```python
from build123d import *

# Parameters (mm, degrees)
F1_DEPTH = 63.5
F2_DEPTH = 3.175
F0_W     = 22.2610938409
F0_H     = 19.05
F3_DEPTH = 25.4
F5_DEPTH = 25.4
F6_R     = 6.35


with BuildPart() as f1:
    # F0 (on Front) → F1 (new body, symmetric)
    with BuildSketch(Plane.XZ):
        Polygon((-41.275, 9.525), (-41.275, -9.525), (41.275, -9.525), (41.275, 9.525), (22.225, 9.525), align=None)
    extrude(amount=F1_DEPTH, both=True)

    # F0 (on Front) → F2 (join, symmetric)
    with BuildSketch(Plane.XZ):
        with BuildLine():
            add(Edge.make_bspline(
                [(-41.275, 9.525), (-34.2779420316, 38.2648594677), (15.5508974567, 65.6356289983), (57.15, 61.9252)],
                knots=[0, 0, 0, 0, 111.5045361635, 111.5045361635, 111.5045361635, 111.5045361635], degree=3))
            Line((-41.275, 9.525), (22.225, 9.525))
            Line((22.225, 9.525), (22.225, 27.0002))
            ThreePointArc((22.225, 27.0002), (32.4542956671, 51.6959043329), (57.15, 61.9252))
        make_face()
    extrude(amount=F2_DEPTH, both=True)

    # F0 (on Front) → F3 (join, symmetric)
    with BuildSketch(Plane.XZ):
        with BuildLine():
            Line((22.225, 9.525), (41.275, 9.525))
            Line((41.275, 9.525), (41.275, 27.0002))
            ThreePointArc((41.275, 27.0002), (45.9246798487, 38.2255201513), (57.15, 42.8752))
            Line((57.15, 42.8752), (60.325, 42.8752))
            Line((60.325, 42.8752), (60.325, 61.9252))
            Line((60.325, 61.9252), (57.15, 61.9252))
            ThreePointArc((57.15, 61.9252), (32.4542956671, 51.6959043329), (22.225, 27.0002))
            Line((22.225, 27.0002), (22.225, 9.525))
        make_face()
        with Locations((71.4555469204, 52.4002)):
            Rectangle(F0_W, F0_H)
    extrude(amount=F3_DEPTH, both=True)

    # F0 (on Front) → F4 (revolve)
    with BuildSketch(Plane.XZ):
        Polygon((82.5860938409, 66.675), (82.5860938409, 61.9252), (82.5860938409, 42.8752), (82.5860938409, 38.1), (111.125, 38.1), (111.125, 66.675), align=None)
    revolve(axis=Axis((82.5860938409, 0, 52.3875), (0, 0, -1)))

    # F0 (on Front) → F5 (join, symmetric)
    with BuildSketch(Plane.XZ):
        with Locations((71.4555469204, 52.4002)):
            Rectangle(F0_W, F0_H)
    extrude(amount=F5_DEPTH, both=True)

    # F6
    f6_edges = [f1.edges().sort_by_distance(p)[0] for p in [
        (41.275, -63.5, 0),
        (-41.275, -63.5, 0),
        (-41.275, 63.5, 0),
        (41.275, 63.5, 0),
    ]]
    fillet(f6_edges, radius=F6_R)


solid = f1.part
```
Read the model definition and answer for the solid it produces. Units are mm, in the model's axes. A direction names the side the tool comes from. Round coordinates to 2 decimals unless told otherwise and drop trailing zeros. Write each loop counter-clockwise with the first axis right and the second up, starting at its lowest first coordinate (ties: lowest second). Pieces come first, ordered by that corner, then holes. Notation, with made-up numbers: M 29.25,15 L 40.25,15 A20 ccw 40.25,40 Z; hole C 83.5,76 d9. An arc over 180 degrees is marked long. One line per item, written item: value.
Q1. Find section C-C on x = 90. Write down the section's boundary in (y, z) (3 decimals).
Data:
outline: M -27.559,38.1 L 27.559,38.1 L 27.559,66.675 L -27.559,66.675 Z
Q2. For a pull along X with two mould halves and no side action, classify faces 1 (the cylindrical face through (32.73, -14.44, 51.97)), 2 (the flat face through (-1, -1, -9.525)), 3 (the flat face through (61, -22, 42.875)) as +X half, -X half, draft (parallel to the pull), parting line (faces both ways), or undercut.
Data:
face 1: -X half
face 2: draft
face 3: undercut
Q3. Straight lines are drawn through the part: line 1 (Z direction, x = -10, y = -58) (3 decimals); line 2 (X direction, y = 26, z = 5) (3 decimals); line 3 (Z direction, x = 93.5, y = 15.5) (3 decimals). For each, find the intervals that lie inside material, in ascending order. Write a range as [from, to].
Data:
line 1: [-9.525, 9.525]
line 2: [-41.275, 41.275]
line 3: [38.1, 66.675]
Q4. Flat-ended cylindrical pins translate along their axes: pin 1 Ø8.5 at (y, z) = (14, 15) entering from -X (3 decimals); pin 2 Ø1.5 at (x, y) = (21.5, -36) entering from +Z (3 decimals); pin 3 Ø2 at (y, z) = (7, 34) entering from +X. Find the tip coordinate at first contact, or state that the pin passes through.
Data:
pin 1: x = 22.225
pin 2: z = 9.525
pin 3: x = 43.44
Q5. Find section B-B on y = 11. Write down the section's boundary in (x, z) (3 decimals), plus the area to 3 significant figures.
Data:
outline: M -41.275,-9.525 L 41.275,-9.525 L 41.275,27 A15.875 cw 56.252,42.85 L 56.252,38.1 L 108.92,38.1 L 108.92,66.675 L 56.252,66.675 L 56.252,61.914 A34.925 ccw 22.225,27 L 22.225,9.525 L -41.275,9.525 Z
area: 4,150 mm2
Q6. Which of the six approach directions +Z, -Z, +X, -X, +Y, -Y give full straight-line access (tool end or side, diameter ignored) to faces 4 (the flat face through (83, 0, 38.1)), 5 (the flat face through (7, 3.175, 31)), 6 (the flat face through (40, -25.4, 36)), 7 (the flat face through (-41.275, -1, 0))?
Data:
face 4: -Z, +X, +Y, -Y
face 5: +Z, -X, +Y
face 6: +Z, -X, -Y
face 7: +Z, -Z, -X, +Y, -Y
Q7. Find section A-A on z = 5.5. Write down the section's boundary in (x, y) (3 decimals), plus the area to 3 significant figures.
Data:
outline: M -41.275,-57.15 A6.35 ccw -34.925,-63.5 L 34.925,-63.5 A6.35 ccw 41.275,-57.15 L 41.275,57.15 A6.35 ccw 34.925,63.5 L -34.925,63.5 A6.35 ccw -41.275,57.15 Z
area: 10,400 mm2
